```python
from build123d import *

# Parameters (mm, degrees)
SKETCH1_W                 = 56.15
SKETCH1_H                 = 48
BOSS_EXTRUDE1_DEPTH       = 5
SKETCH2_W                 = 10
SKETCH2_H                 = 48
BOSS_EXTRUDE2_DEPTH       = 73.5
SKETCH3_W                 = 24
SKETCH3_H                 = 10
BOSS_EXTRUDE3_DEPTH       = 20
SKETCH19_W                = 24
SKETCH19_H                = 10
BOSS_EXTRUDE5_DEPTH       = 20
FILLET1_R                 = 10
F_1_0MM_DOWEL_HOLE1_D     = 5.5
F_1_0MM_DOWEL_HOLE1_DEPTH = 10
FILLET2_R                 = 5
M6_CLEARANCE_HOLE1_D      = 16.15
CHAMFER2_SIZE             = 4
SKETCH14_W                = 17
SKETCH14_H                = 5
BOSS_EXTRUDE4_DEPTH       = 20
CHAMFER3_SIZE             = 10
FILLET3_R                 = 2
M2_START                  = -15.5
M2_CLEARANCE_SLOT1_DEPTH  = 5
RIB1_REACH                = 114.898
SKETCH20_WALL_W           = 249.008442536
SKETCH20_WALL_H           = 4
RIB2_REACH                = 104.107
SKETCH21_WALL_W           = 227.427527126
SKETCH21_WALL_H           = 4
RIB10_REACH               = 104.107
SKETCH23_WALL_W           = 221.21432369
SKETCH23_WALL_H           = 4


# Read off the part's stored shape, not the designer's step: M2 Clearance Slot1
with BuildPart() as part:
    # Sketch1 → Boss-Extrude1 (new body)
    with BuildSketch(Plane(origin=(0, 0, 0), x_dir=(1, 0, 0), z_dir=(0, 1, 0))):
        with Locations((4.075, 0)):
            Rectangle(SKETCH1_W, SKETCH1_H)
    extrude(amount=BOSS_EXTRUDE1_DEPTH)

    # Sketch2 → Boss-Extrude2 (add)
    with BuildSketch(Plane.XZ):
        with Locations((27.15, 0)):
            Rectangle(SKETCH2_W, SKETCH2_H)
    extrude(amount=BOSS_EXTRUDE2_DEPTH)

    # Sketch3 → Boss-Extrude3 (add)
    with BuildSketch(Plane(origin=(32.15, 0, 0), x_dir=(0, 0, -1), z_dir=(1, 0, 0))):
        with Locations((12, -68.5)):
            Rectangle(SKETCH3_W, SKETCH3_H)
    extrude(amount=BOSS_EXTRUDE3_DEPTH)

    # Sketch19 → Boss-Extrude5 (add)
    with BuildSketch(Plane(origin=(22.15, 0, -25.5), x_dir=(0, 0, 1), z_dir=(-1, 0, 0))):
        with Locations((37.5, -68.5)):
            Rectangle(SKETCH19_W, SKETCH19_H)
    extrude(amount=BOSS_EXTRUDE5_DEPTH)

    # Fillet1
    fillet1_edges = [part.edges().sort_by_distance(p)[0] for p in [
        (-24, 2.5, -24),
        (-24, 2.5, 24),
    ]]
    fillet(fillet1_edges, radius=FILLET1_R)

    # Ø1.0mm Dowel Hole1
    with Locations(Plane(origin=(0, -63.5, 0), x_dir=(1, 0, 0), z_dir=(0, 1, 0))):
        with Locations((42.15, 12), (12.15, -12)):
            Hole(F_1_0MM_DOWEL_HOLE1_D / 2, depth=F_1_0MM_DOWEL_HOLE1_DEPTH)

    # Fillet2
    fillet2_edges = [part.edges().sort_by_distance(p)[0] for p in [
        (52.15, -68.5, 0),
        (52.15, -68.5, -24),
        (2.15, -68.5, 0),
        (2.15, -68.5, 24),
    ]]
    fillet(fillet2_edges, radius=FILLET2_R)

    # M6 Clearance Hole1 (through all)
    with Locations(Plane(origin=(0, 5, 0), x_dir=(1, 0, 0), z_dir=(0, 1, 0))):
        with Locations((-7.85, 0)):
            Hole(M6_CLEARANCE_HOLE1_D / 2)

    # Chamfer2
    chamfer2_edges = [part.edges().sort_by_distance(p)[0] for p in [
        (32.15, 5, 0),
    ]]
    chamfer(chamfer2_edges, length=CHAMFER2_SIZE)

    # Sketch14 → Boss-Extrude4 (add)
    with BuildSketch(Plane.XY.offset(24)):
        with Locations((30.65, -13)):
            Rectangle(SKETCH14_W, SKETCH14_H)
    extrude(amount=BOSS_EXTRUDE4_DEPTH)

    # Chamfer3
    # the kernel refuses this chamfer: 10 mm, written as the material it adds along each edge
    with BuildSketch(Plane(origin=(32.15, -10.5, 24), x_dir=(-0.027495876610586317, 0, -0.9996219169112968), z_dir=(0, -1, 0))) as chamfer3_piece_1_section:
        Polygon((CHAMFER3_SIZE * 0.999621916911, CHAMFER3_SIZE * 0.0274958766106), (-CHAMFER3_SIZE * 0.0274958766106, CHAMFER3_SIZE * 0.999621916911), (0, 0), align=None)
    chamfer3_piece_1 = extrude(amount=5, mode=Mode.PRIVATE)
    chamfer3_piece_1 = split(chamfer3_piece_1, bisect_by=Plane(origin=(39.15, -13, 20.435897436), z_dir=(-1, 0, 0)), keep=Keep.TOP, mode=Mode.PRIVATE)
    add(chamfer3_piece_1)

    # Fillet3
    fillet3_edges = [part.edges().sort_by_distance(p)[0] for p in [
        (27.15, -15.5, 24),
        (22.15, -13, 44),
        (39.15, -13, 44),
        (32.15, -15.5, 19),
    ]]
    fillet(fillet3_edges, radius=FILLET3_R)

    # M2 Clearance Slot1 outline → M2 Clearance Slot1 (cut)
    with BuildSketch(Plane(origin=(0, 0, 0), x_dir=(1, 0, 0), z_dir=(0, 1, 0)).offset(M2_START)):
        with BuildLine():
            Line((34.65, -27.8), (29.65, -27.8))
            ThreePointArc((29.65, -27.8), (28.45, -29), (29.65, -30.2))
            Line((29.65, -30.2), (34.65, -30.2))
            ThreePointArc((34.65, -30.2), (35.85, -29), (34.65, -27.8))
        make_face()
        with BuildLine():
            Line((34.65, -37.3), (29.65, -37.3))
            ThreePointArc((29.65, -37.3), (28.45, -38.5), (29.65, -39.7))
            Line((29.65, -39.7), (34.65, -39.7))
            ThreePointArc((34.65, -39.7), (35.85, -38.5), (34.65, -37.3))
        make_face()
    extrude(amount=M2_CLEARANCE_SLOT1_DEPTH, mode=Mode.SUBTRACT)

    # Sketch20 wall → Rib1 (add, up to next)
    with BuildSketch(Plane(origin=(39.65, -56, -24), x_dir=(-0.707106781187, 0.707106781187, 0), z_dir=(0.707106781187, 0.707106781187, 0)), mode=Mode.PRIVATE) as rib1_sk1:
        with Locations((0, 2)):
            Rectangle(SKETCH20_WALL_W, SKETCH20_WALL_H)
    rib1_tool1 = extrude(rib1_sk1.sketch, amount=-RIB1_REACH, mode=Mode.PRIVATE) - part.part
    rib1 = rib1_tool1.solids().sort_by_distance((39.65, -56, -24))[0]
    add(rib1)

    # Sketch21 wall → Rib2 (add, up to next)
    with BuildSketch(Plane(origin=(14.65, -56, 24), x_dir=(0.707106781187, 0.707106781187, 0), z_dir=(-0.707106781187, 0.707106781187, 0)), mode=Mode.PRIVATE) as rib2_sk1:
        with Locations((0, 2)):
            Rectangle(SKETCH21_WALL_W, SKETCH21_WALL_H)
    rib2_tool1 = extrude(rib2_sk1.sketch, amount=-RIB2_REACH, mode=Mode.PRIVATE) - part.part
    rib2 = rib2_tool1.solids().sort_by_distance((14.65, -56, 24))[0]
    add(rib2)

    # Sketch23 wall → Rib10 (add, up to next)
    with BuildSketch(Plane(origin=(16.846699141, -5.303300859, 24), x_dir=(-0.707106781187, 0.707106781187, 0), z_dir=(-0.707106781187, -0.707106781187, 0)), mode=Mode.PRIVATE) as rib10_sk1:
        with Locations((0, 2)):
            Rectangle(SKETCH23_WALL_W, SKETCH23_WALL_H)
    rib10_tool1 = extrude(rib10_sk1.sketch, amount=-RIB10_REACH, mode=Mode.PRIVATE) - part.part
    rib10 = rib10_tool1.solids().sort_by_distance((16.846699141, -5.303300859, 24))[0]
    add(rib10)

    # Mirror1: Rib2 across plane
    add(rib2.mirror(Plane(origin=(2.15, -63.5, 12), x_dir=(1, 0, 0), z_dir=(0, 0, 1))))

    # Mirror2: Rib1 across plane
    add(rib1.mirror(Plane(origin=(52.15, -63.5, -12), x_dir=(1, 0, 0), z_dir=(0, 0, -1))))

    # Mirror3: Rib10 across plane
    add(rib10.mirror(Plane.XY))


solid = part.part
```
Could you check a few things on this model? Use its own coordinates, in mm. A direction names the side the tool comes from. Coordinates: 2 decimals unless noted, no trailing zeros. Loops run counter-clockwise (first coordinate to the right, second up) from the corner with the lowest first, then second, coordinate; pieces in that order, holes last.
1) Will these pins go through, and if not, where does the flat tip stop? pin 1 Ø5 at (x, z) = (32.5, 30) entering from +Y; pin 2 Ø16.5 at (x, y) = (18, -56.5) entering from +Z; pin 3 Ø8 at (y, z) = (-22, -10) entering from +X; pin 4 Ø2.5 at (x, y) = (33, -12) entering from -Z.
Reported:
pin 1: stops at y = -10.5
pin 2: stops at z = 24
pin 3: stops at x = 32.15
pin 4: stops at z = -24
2) Please list where these lines run through material, in increasing order: line 1 along X through (y, z) = (-70, 12); line 2 along Y through (x, z) = (19.5, 4.5); line 3 along Z through (x, y) = (12.15, -66.75).
Reported:
line 1: x = 2.15 to 9.4, 14.9 to 32.15
line 2: y = -73.5 to -63.5, 0 to 5
line 3: z = 0 to 9.25, 14.75 to 24
3) Imagine slicing it at D-D (y = -61). List the corners of the cut face in (x, z) for me, and give its area (3 significant figures).
Reported:
outline: (9.65, 0) - (22.15, 0) - (22.15, -24) - (44.65, -24) - (44.65, -20) - (32.15, -20) - (32.15, -4) - (44.65, -4) - (44.65, 0) - (32.15, 0) - (32.15, 24) - (9.65, 24) - (9.65, 20) - (22.15, 20) - (22.15, 4) - (9.65, 4) - close
area: 680 mm2
4) Which directions (+Z, -Z, +X, -X, +Y, -Y) give clear straight access to the entire face, cutting with the end or side of a thin tool? Please do faces 4 (the face through (32, -13, 30.2)), 5 (the face through (2.15, -68, 12)), 6 (the face through (16.921, -5.378, 21.972)), 7 (the face through (19, -3, 20)).
Reported:
face 4: +Y, -Y
face 5: +Z, -Z, -X, -Y
face 6: +Z, -Z, -X
face 7: -X
5) Thinking about a two-plate mould opening in Y: for faces 1 (the face through (16.921, -5.378, -21.972)), 2 (the face through (17, -59, 4)), 3 (the face through (35.85, -13.04, 29.03)), which applies, released by +Y, released by -Y, zero draft, split by the parting line, or undercut?
Reported:
face 1: released by -Y
face 2: undercut
face 3: zero draft
6) Imagine slicing it at C-C (x = 13). List the corners of the cut face in (y, z) for me, and give its area (3 significant figures).
Reported:
outline: (-73.5, 0) - (-57.65, 0) - (-57.65, 4) - (-63.5, 4) - (-63.5, 9.38) - (-73.5, 9.38) - close; (-73.5, 14.62) - (-63.5, 14.62) - (-63.5, 20) - (-57.65, 20) - (-57.65, 24) - (-73.5, 24) - close; (-1.46, -24) - (5, -24) - (5, 24) - (-1.46, 24) - (-1.46, 20) - (0, 20) - (0, -20) - (-1.46, -20) - close
area: 486 mm2
7) Imagine slicing it at B-B (y = -12.5). List the corners of the cut face in (x, z) for me.
Reported:
outline: (22.15, -24) - (32.15, -24) - (32.15, 14) - (39.15, 21) - (39.15, 42) arc R2 ccw to (37.15, 44) - (24.15, 44) arc R2 ccw to (22.15, 42) - close; hole (29.65, 27.8) - (34.65, 27.8) arc R1.2 ccw to (34.65, 30.2) - (29.65, 30.2) arc R1.2 ccw to start; hole (29.65, 37.3) - (34.65, 37.3) arc R1.2 ccw to (34.65, 39.7) - (29.65, 39.7) arc R1.2 ccw to start
8) Imagine slicing it at A-A (x = -7.85). List the corners of the cut face in (y, z) for me (3 decimals), and give its area (3 significant figures).
Reported:
outline: (0, -24) - (5, -24) - (5, -8.075) - (0, -8.075) - close; (0, 8.075) - (5, 8.075) - (5, 24) - (0, 24) - close
area: 159 mm2
